from build123d import *

# Parameters (mm, degrees)
SKETCH2_W           = 96.52
SKETCH2_H           = 66.04
BOSS_EXTRUDE1_DEPTH = 17.78
SKETCH3_W           = 96.52
SKETCH3_H           = 5.588
BOSS_EXTRUDE2_DEPTH = 12.7
SKETCH4_W           = 86.6394
SKETCH4_H           = 9.525
SKETCH4_W_2         = 76.2
SKETCH4_H_2         = 3.175
CUT_EXTRUDE1_DEPTH  = 60.452
SKETCH5_W           = 96.52
SKETCH5_H           = 5.588
BOSS_EXTRUDE3_DEPTH = 12.7
SKETCH6_R           = 2.413
SKETCH6_R_2         = 3.81
CUT_EXTRUDE2_DEPTH  = 6.588
FILLET1_R           = 1.27
FILLET2_R           = 1.27
FILLET3_R           = 1.27


with BuildPart() as part:
    # Sketch2 → Boss-Extrude1 (new body)
    with BuildSketch(Plane.XY):
        with Locations((48.26, 33.02)):
            Rectangle(SKETCH2_W, SKETCH2_H)
    extrude(amount=BOSS_EXTRUDE1_DEPTH)

    # Sketch3 → Boss-Extrude2 (add)
    with BuildSketch(Plane.XY.offset(17.78)):
        with Locations((48.26, 2.794)):
            Rectangle(SKETCH3_W, SKETCH3_H)
    extrude(amount=BOSS_EXTRUDE2_DEPTH)

    # Sketch4 → Cut-Extrude1 (cut)
    with BuildSketch(Plane(origin=(0, 66.04, 0), x_dir=(1, 0, 0), z_dir=(0, 1, 0))):
        with Locations((48.26, -9.8425)):
            Rectangle(SKETCH4_W, SKETCH4_H)
        with Locations((48.26, -16.1925)):
            Rectangle(SKETCH4_W_2, SKETCH4_H_2)
    extrude(amount=-CUT_EXTRUDE1_DEPTH, mode=Mode.SUBTRACT)

    # Sketch5 → Boss-Extrude3 (add)
    with BuildSketch(Plane(origin=(0, 0, 0), x_dir=(-1, 0, 0), z_dir=(0, 0, -1))):
        with Locations((-48.26, 2.794)):
            Rectangle(SKETCH5_W, SKETCH5_H)
    extrude(amount=BOSS_EXTRUDE3_DEPTH)

    # Sketch6 → Cut-Extrude2 (cut, through all)
    with BuildSketch(Plane(origin=(0, 5.588, 0), x_dir=(1, 0, 0), z_dir=(0, 1, 0))):
        with Locations((10.16, 6.35)):
            Circle(SKETCH6_R)
        with Locations((22.86, 6.35)):
            Circle(SKETCH6_R)
        with Locations((35.56, 6.35)):
            Circle(SKETCH6_R)
        with Locations((48.26, 6.35)):
            Circle(SKETCH6_R)
        with Locations((60.96, 6.35)):
            Circle(SKETCH6_R)
        with Locations((73.66, 6.35)):
            Circle(SKETCH6_R)
        with Locations((86.36, 6.35)):
            Circle(SKETCH6_R)
        with Locations((10.16, -22.86)):
            Circle(SKETCH6_R_2)
        with Locations((25.4, -22.86)):
            Circle(SKETCH6_R_2)
        with Locations((40.64, -22.86)):
            Circle(SKETCH6_R_2)
        with Locations((55.88, -22.86)):
            Circle(SKETCH6_R_2)
        with Locations((71.12, -22.86)):
            Circle(SKETCH6_R_2)
        with Locations((86.36, -22.86)):
            Circle(SKETCH6_R_2)
    extrude(amount=-CUT_EXTRUDE2_DEPTH, mode=Mode.SUBTRACT)

    # Fillet1
    fillet1_edges = [part.edges().sort_by_distance(p)[0] for p in [
        (91.44, 66.04, 17.78),
        (5.08, 66.04, 17.78),
        (91.5797, 66.04, 9.8425),
        (48.26, 66.04, 5.08),
        (4.9403, 66.04, 9.8425),
        (7.55015, 66.04, 14.605),
        (10.16, 66.04, 16.1925),
        (88.96985, 66.04, 14.605),
        (86.36, 66.04, 16.1925),
        (48.26, 66.04, 0),
        (0, 66.04, 8.89),
        (96.52, 66.04, 8.89),
    ]]
    fillet(fillet1_edges, radius=FILLET1_R)

    # Fillet2
    fillet2_edges = [part.edges().sort_by_distance(p)[0] for p in [
        (0, 5.588, 24.13),
        (96.52, 5.588, 24.13),
        (48.26, 5.588, 30.48),
        (96.52, 5.588, -6.35),
        (0, 5.588, -6.35),
        (48.26, 5.588, -12.7),
    ]]
    fillet(fillet2_edges, radius=FILLET2_R)

    # Fillet3
    fillet3_edges = [part.edges().sort_by_distance(p)[0] for p in [
        (48.26, 0, 30.48),
        (48.26, 0, -12.7),
        (96.52, 0, 8.89),
        (0, 0, 8.89),
    ]]
    fillet(fillet3_edges, radius=FILLET3_R)


solid = part.part
Can you work these out from the model? Positions are in its coordinate system, mm. A direction names the side the tool comes from. Round coordinates to 2 decimals unless told otherwise and drop trailing zeros. Loops run counter-clockwise (first coordinate to the right, second up) from the corner with the lowest first, then second, coordinate; pieces in that order, holes last. Notation, with made-up numbers: (0.25, 1) - (15.25, 1) arc R29 cw to (15.25, 22) - close; hole circle Ø5 at (9.5, 61). An arc over 180 degrees is marked (long way). Answer in a Markdown table with one row per item. Add a question column.
Q1. I need wall thicknesses on L1, parallel to Z at x = 10.16, y = 2.1; L2, parallel to X at y = 49, z = 10.5; L3, parallel to Z at x = 7, y = 26 (3 decimals). Which ranges of each line are inside material? Lowest first, please.
Q2. I want a section at C-C on y = 43. List the corners of the cut face in (x, z) for me (3 decimals).
Q3. Which directions (+Z, -Z, +X, -X, +Y, -Y) give clear straight access to the entire face, cutting with the end or side of a thin tool? Please do faces 1 (the flat face through (91.58, 36, 10)), 2 (the cylindrical face through (88.662, 2.833, -7.075)), 3 (the flat face through (10.16, 36, 16)).
Q4. I want a section at B-B on z = 22.86. Count the separate pieces of the cut face and the enclosed holes in it, and give its area (3 significant figures).
Q5. I want a section at A-A on x = 55.88. List the corners of the cut face in (y, z) for me, and give its area (3 significant figures).
Q6. We'd pull the mould along X, two halves only. Please class faces 4 (the flat face through (0, 33, 9)), 5 (the cylindrical face through (71.25, 2.83, -6.46)), 6 (the flat face through (49, 5.588, -3)): pulls with the +X half, pulls with the -X half, needs draft (parallel to the pull), parting line crosses it, or undercut.
Q7. For pin 1 Ø12 at (x, z) = (71.12, 22.86) entering from +Y; pin 2 Ø12 at (x, z) = (86.36, 22.86) entering from +Y; pin 3 Ø5.5 at (x, y) = (89, 41.5) entering from -Z; pin 4 Ø6 at (x, z) = (55.88, 22.86) entering from +Y, each with a flat end and sliding along its axis, tell me the tip position at first contact or that it passes through.
A:
| question | item | result |
|---|---|---|
| 1 | L1 | -12.7 to -8.76, -3.94 to 19.05, 26.67 to 30.48 |
| 1 | L2 | 0 to 4.94, 91.58 to 96.52 |
| 1 | L3 | 0 to 5.08, 14.605 to 17.78 |
| 2 | outline | (0, 0) - (96.52, 0) - (96.52, 17.78) - (86.36, 17.78) - (86.36, 14.605) - (91.58, 14.605) - (91.58, 5.08) - (4.94, 5.08) - (4.94, 14.605) - (10.16, 14.605) - (10.16, 17.78) - (0, 17.78) - close |
| 3 | face 1 | +Y |
| 3 | face 2 | +Y, -Y |
| 3 | face 3 | +Z, +Y |
| 4 | separate pieces | 7 |
| 4 | enclosed holes | 0 |
| 4 | area | 282 mm^2 |
| 5 | outline | (0, -11.43) arc R1.27 ccw to (1.27, -12.7) - (4.32, -12.7) arc R1.27 ccw to (5.59, -11.43) - (5.59, 0) - (64.77, 0) arc R1.27 ccw to (66.04, 1.27) - (66.04, 3.81) arc R1.27 ccw to (64.77, 5.08) - (5.59, 5.08) - (5.59, 19.05) - (0, 19.05) - close; (0, 26.67) - (5.59, 26.67) - (5.59, 29.21) arc R1.27 ccw to (4.32, 30.48) - (1.27, 30.48) arc R1.27 ccw to (0, 29.21) - close |
| 5 | area | 504 mm^2 |
| 6 | face 4 | pulls with the -X half |
| 6 | face 5 | undercut |
| 6 | face 6 | needs draft |
| 7 | pin 1 | y = 5.59 |
| 7 | pin 2 | y = 65.97 |
| 7 | pin 3 | z = 0 |
| 7 | pin 4 | through |
